The listing builds one solid part. Answer for the finished solid, in the listing's coordinates (mm). Face numbers are marked on the shaded views. A direction names the side the tool comes from. Round coordinates to 2 decimals unless told otherwise and drop trailing zeros. Loops run counter-clockwise (first coordinate to the right, second up) from the corner with the lowest first, then second, coordinate; pieces in that order, holes last. Notation, with made-up numbers: (2, 79) -> (54, 79) arc R24 cw to (54, 95) -> close; hole circle Ø2 at (69.25, 7.5). An arc over 180 degrees is marked (long way). One line per question, with ' | ' between items.
from build123d import *

# Parameters (mm, degrees)
SKETCH1_W           = 800
SKETCH1_H           = 495
BOSS_EXTRUDE1_DEPTH = 9
FILLET1_R           = 8
FILLET2_R           = 1
SKETCH2_W           = 775
SKETCH2_H           = 472
BOSS_EXTRUDE2_DEPTH = 4
SKETCH3_W           = 170
SKETCH3_H           = 380
BOSS_EXTRUDE3_DEPTH = 130
SKETCH4_W           = 360
SKETCH4_H           = 450
BOSS_EXTRUDE4_DEPTH = 210


with BuildPart() as part:
    # Sketch1 → Boss-Extrude1 (new body)
    with BuildSketch(Plane(origin=(0, 0, 0), x_dir=(1, 0, 0), z_dir=(0, 1, 0))):
        Rectangle(SKETCH1_W, SKETCH1_H)
    extrude(amount=-BOSS_EXTRUDE1_DEPTH)

    # Fillet1
    fillet1_edges = [part.edges().sort_by_distance(p)[0] for p in [
        (-400, -4.5, -247.5),
        (400, -4.5, -247.5),
        (400, -4.5, 247.5),
        (-400, -4.5, 247.5),
    ]]
    fillet(fillet1_edges, radius=FILLET1_R)

    # Fillet2
    fillet2_edges = [part.edges().sort_by_distance(p)[0] for p in [
        (400, 0, 0),
        (-400, 0, 0),
        (0, 0, 247.5),
        (0, 0, -247.5),
        (397.656854249, 0, 245.156854249),
        (-397.656854249, 0, 245.156854249),
        (-397.656854249, 0, -245.156854249),
        (397.656854249, 0, -245.156854249),
    ]]
    fillet(fillet2_edges, radius=FILLET2_R)

    # Sketch2 → Boss-Extrude2 (add)
    with BuildSketch(Plane.XZ.offset(9)):
        Rectangle(SKETCH2_W, SKETCH2_H)
    extrude(amount=BOSS_EXTRUDE2_DEPTH)

    # Sketch3 → Boss-Extrude3 (add)
    with BuildSketch(Plane(origin=(0, 0, 0), x_dir=(1, 0, 0), z_dir=(0, 1, 0))):
        with Locations((-84, 0)):
            Rectangle(SKETCH3_W, SKETCH3_H)
    extrude(amount=-BOSS_EXTRUDE3_DEPTH)

    # Sketch4 → Boss-Extrude4 (add)
    with BuildSketch(Plane(origin=(0, 0, 0), x_dir=(1, 0, 0), z_dir=(0, 1, 0))):
        with Locations((189, 0)):
            Rectangle(SKETCH4_W, SKETCH4_H)
    extrude(amount=-BOSS_EXTRUDE4_DEPTH)


solid = part.part
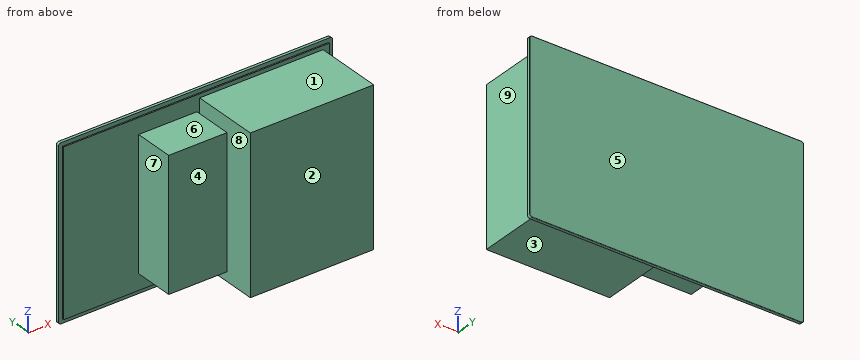
Q1. For the marked faces 1, 2, 3, 4 and 5, determine the directions among +Z, -Z, +X, -X, +Y, -Y from which every point of the face is accessible in a straight line to the end or side of a thin tool.
Numbers:
face 1: +Z, +X, -X, -Y | face 2: +Z, -Z, +X, -X, -Y | face 3: -Z, +X, -X, -Y | face 4: +Z, -Z, -X, -Y | face 5: +Z, -Z, +X, -X, +Y
Q2. A cutting plane is placed at A-A on z = -203.5. Give the vertices of the cut face in (x, y), plus the area to 3 significant figures.
Numbers:
outline: (-400, -9) -> (-387.5, -9) -> (-387.5, -13) -> (9, -13) -> (9, -210) -> (369, -210) -> (369, -13) -> (387.5, -13) -> (387.5, -9) -> (400, -9) -> (400, -1) arc R1 ccw to (399, 0) -> (-399, 0) arc R1 ccw to (-400, -1) -> close | area: 81,200 mm^2
Q3. Given pin 1 Ø2 at (y, z) = (-139.5, -166) entering from +X; pin 2 Ø3 at (x, y) = (-61, -122) entering from -Z; pin 3 Ø4 at (x, y) = (213, -100) entering from -Z, each flat-ended and moving along its own axis, determine where each tip first touches the part or whether it passes through.
Numbers:
pin 1: x = 369 | pin 2: z = -190 | pin 3: z = -225
Q4. Find the intervals of material crossed by line 1 (X direction, y = -115, z = -183.5); line 2 (X direction, y = -177, z = 5.5); line 3 (Y direction, x = -41, z = 204), in increasing order. Write a range as from..to.
Numbers:
line 1: -169..1, 9..369 | line 2: 9..369 | line 3: -13..0
Q5. A cutting plane is placed at B-B on x = 48. Give the vertices of the cut face in (y, z).
Numbers:
outline: (-210, -225) -> (-13, -225) -> (-13, -236) -> (-9, -236) -> (-9, -247.5) -> (-1, -247.5) arc R1 ccw to (0, -246.5) -> (0, 246.5) arc R1 ccw to (-1, 247.5) -> (-9, 247.5) -> (-9, 236) -> (-13, 236) -> (-13, 225) -> (-210, 225) -> close
Q6. For a pull along X with two mould halves and no side action, classify the marked faces 6, 7, 8 and 9 as pulls with the +X half, pulls with the -X half, needs draft (parallel to the pull), parting line crosses it, or undercut.
Numbers:
face 6: needs draft | face 7: pulls with the -X half | face 8: undercut | face 9: pulls with the +X half
Q7. A cutting plane is placed at D-D on z = 119.5. Give the vertices of the cut face in (x, y).
Numbers:
outline: (-400, -9) -> (-387.5, -9) -> (-387.5, -13) -> (-169, -13) -> (-169, -130) -> (1, -130) -> (1, -13) -> (9, -13) -> (9, -210) -> (369, -210) -> (369, -13) -> (387.5, -13) -> (387.5, -9) -> (400, -9) -> (400, -1) arc R1 ccw to (399, 0) -> (-399, 0) arc R1 ccw to (-400, -1) -> close
Q8. A cutting plane is placed at C-C on y = -44. Give the vertices of the cut face in (x, z), plus the area to 3 significant figures.
Numbers:
outline: (-169, -190) -> (1, -190) -> (1, 190) -> (-169, 190) -> close; (9, -225) -> (369, -225) -> (369, 225) -> (9, 225) -> close | area: 227,000 mm^2
